```python
from build123d import *

# Parameters (mm, degrees)
F0_R     = 12.7
F1_DEPTH = 12.7
F2_R     = 3.175
F3_DEPTH = 101.6
F4_R     = 12.6988546774
F5_DEPTH = 12.7
F6_R     = 5.08


with BuildPart() as f1:
    # F0 (on Top) → F1 (new body)
    with BuildSketch(Plane.XY):
        Circle(F0_R)
    extrude(amount=F1_DEPTH)

    # F2 (on face) → F3 (join)
    with BuildSketch(Plane.XY.offset(12.7)):
        Circle(F2_R)
    extrude(amount=F3_DEPTH)

    # F4 (on face) → F5 (join)
    with BuildSketch(Plane.XY.offset(114.3)):
        Circle(F4_R)
    extrude(amount=F5_DEPTH)

    # F6
    f6_edges = [f1.edges().sort_by_distance(p)[0] for p in [
        (-12.7, 0, 12.7),
        (-12.7, 0, 0),
        (-12.698855, 0, 127),
        (-12.698855, 0, 114.3),
    ]]
    fillet(f6_edges, radius=F6_R)


with BuildPart() as f1_1:
    # F7: moved
    add(f1.part.moved(Location((0, 0, -52.324))))


solid = f1_1.part
```
CAD build for the part. Positions are in the model's coordinates, mm. A direction names the side the tool comes from. Coordinates: 2 decimals unless noted, no trailing zeros. Write each loop counter-clockwise with the first axis right and the second up, starting at its lowest first coordinate (ties: lowest second). Pieces come first, ordered by that corner, then holes. Notation, with made-up numbers: (57.25, 78.5) -> (70.25, 78.5) arc R26 cw to (70.25, 102.5) -> close; hole circle Ø10 at (43, -12.75). An arc over 180 degrees is marked (long way). Return JSON: item names as keys, results as strings. Group by question number.
Q1. Cut at A-A, the plane x = 0. Give the cut face in (y, z) (3 decimals).
Q2. Drill centre lines: line 1 (Z direction, x = -3, y = 4.25); line 2 (Z direction, x = 3, y = 10.25); line 3 (Y direction, x = 0, z = -22) (3 decimals). Where is each one in solid material? Low to high.
Q3. Pull direction Z, two halves, no side cores. Call faces 1 (the face through (6.827, 10.708, 68.308)), 2 (the face through (0, 0, -52.324)), 3 (the face through (0, 0, 74.676)), 4 (the face through (2, -3, 61.976)): released by +Z, released by -Z, zero draft, split by the parting line, or undercut.
Q4. Flat gauge pins, fed straight in: pin 1 (12 mm diameter, centred on y = 1.5, z = 44, fed in from -X) (3 decimals); pin 2 (5 mm diameter, centred on x = -4, z = 21.5, fed in from -Y); pin 3 (6 mm diameter, centred on x = 9.5, y = -8.5, fed in from -Z). Where does each tip first touch, or does it go through?
Q5. Cut at C-C, the plane z = 7. Give the cut face in (x, y) (3 decimals).
Q6. Which spindle directions (+Z, -Z, +X, -X, +Y, -Y) get a long thin tool onto all of the face, cutting with end or side? Do faces 5 (the face through (3, -2, -39.624)), 6 (the face through (-2.75, -12.4, -45.99)). Say none if no direction does.
Returned:
{
 "1": {"outline": "(-12.7, -47.244) arc R5.08 ccw to (-7.62, -52.324) -> (7.62, -52.324) arc R5.08 ccw to (12.7, -47.244) -> (12.7, -44.704) arc R5.08 ccw to (7.62, -39.624) -> (3.175, -39.624) -> (3.175, 61.976) -> (7.619, 61.976) arc R5.08 ccw to (12.699, 67.056) -> (12.699, 69.596) arc R5.08 ccw to (7.619, 74.676) -> (-7.619, 74.676) arc R5.08 ccw to (-12.699, 69.596) -> (-12.699, 67.056) arc R5.08 ccw to (-7.619, 61.976) -> (-3.175, 61.976) -> (-3.175, -39.624) -> (-7.62, -39.624) arc R5.08 ccw to (-12.7, -44.704) -> close"},
 "2": {"line 1": "z = -52.32 to -39.62, 61.98 to 74.68", "line 2": "z = -51.3 to -40.65, 63 to 73.65", "line 3": "y = -3.175 to 3.175"},
 "3": {"face 1": "zero draft", "face 2": "released by -Z", "face 3": "released by +Z", "face 4": "undercut"},
 "4": {"pin 1": "stops at x = -3.175", "pin 2": "stops at y = -2.8", "pin 3": "stops at z = -51.86"},
 "5": {"outline": "circle Ø6.35 at (0, 0)"},
 "6": {"face 5": "none", "face 6": "+Z, -Z"}
}
